Verification items for the finished model (mm, model axes). A direction names the side the tool comes from. Give positions to 0.01 mm unless a question says otherwise; leave off trailing zeros. Write each loop counter-clockwise with the first axis right and the second up, starting at its lowest first coordinate (ties: lowest second). Pieces come first, ordered by that corner, then holes. Notation, with made-up numbers: M 87.25,10.5 L 144.25,10.5 A16 cw 144.25,25.5 Z; hole C -16.5,54 d11. An arc over 180 degrees is marked long. Answer as a JSON object with one key per item and string values.
```python
from build123d import *

# Parameters (mm, degrees)
CROQUIS1_W              = 55.5
CROQUIS1_H              = 20
CROQUIS1_R              = 1.000000224
CROQUIS1_R_2            = 1.000000066
CROQUIS1_R_3            = 1.500000028
CROQUIS1_R_4            = 0.999999891
CROQUIS1_R_5            = 0.999999587
CROQUIS1_W_2            = 15
CROQUIS1_H_2            = 10
SALIENTE_EXTRUIR1_DEPTH = 4.1
CROQUIS2_W              = 42
CROQUIS2_H              = 20
CROQUIS2_R              = 1.500000028
CROQUIS2_W_2            = 15
CROQUIS2_H_2            = 10
SALIENTE_EXTRUIR2_DEPTH = 5.4
CROQUIS3_R              = 10.033223334
CROQUIS3_R_2            = 1.500000028
SALIENTE_EXTRUIR3_DEPTH = 3.5
CROQUIS4_R              = 5
CROQUIS4_R_2            = 1.500000028
SALIENTE_EXTRUIR4_DEPTH = 3.4


with BuildPart() as part:
    # Croquis1 → Saliente-Extruir1 (new body)
    with BuildSketch(Plane(origin=(0, 0, 0), x_dir=(1, 0, 0), z_dir=(0, 1, 0))):
        with Locations((-0.49546198, -0.123865495)):
            Rectangle(CROQUIS1_W, CROQUIS1_H)
        with Locations((-24.995460911, 4.876134086)):
            Circle(CROQUIS1_R, mode=Mode.SUBTRACT)
        with Locations((-24.995461734, -5.123865495)):
            Circle(CROQUIS1_R_2, mode=Mode.SUBTRACT)
        with Locations((9.504538064, -0.123865505)):
            Circle(CROQUIS1_R_3, mode=Mode.SUBTRACT)
        with Locations((24.004538739, 4.876134747)):
            Circle(CROQUIS1_R_4, mode=Mode.SUBTRACT)
        with Locations((24.004537606, -5.123865416)):
            Circle(CROQUIS1_R_5, mode=Mode.SUBTRACT)
        with Locations((-9.99546198, -0.123865495)):
            Rectangle(CROQUIS1_W_2, CROQUIS1_H_2, mode=Mode.SUBTRACT)
    extrude(amount=SALIENTE_EXTRUIR1_DEPTH)

    # Croquis2 → Saliente-Extruir2 (add)
    with BuildSketch(Plane(origin=(0, 4.1, 0), x_dir=(1, 0, 0), z_dir=(0, 1, 0))):
        with Locations((-0.49546198, -0.123865495)):
            Rectangle(CROQUIS2_W, CROQUIS2_H)
        with Locations((9.504538064, -0.123865505)):
            Circle(CROQUIS2_R, mode=Mode.SUBTRACT)
        with Locations((-9.99546198, -0.123865495)):
            Rectangle(CROQUIS2_W_2, CROQUIS2_H_2, mode=Mode.SUBTRACT)
    extrude(amount=SALIENTE_EXTRUIR2_DEPTH)

    # Croquis3 → Saliente-Extruir3 (add)
    with BuildSketch(Plane(origin=(0, 9.5, 0), x_dir=(1, 0, 0), z_dir=(0, 1, 0))):
        with Locations((9.504538064, -0.123865505)):
            Circle(CROQUIS3_R)
        with Locations((9.504538064, -0.123865505)):
            Circle(CROQUIS3_R_2, mode=Mode.SUBTRACT)
    extrude(amount=SALIENTE_EXTRUIR3_DEPTH)

    # Croquis4 → Saliente-Extruir4 (add)
    with BuildSketch(Plane(origin=(0, 13, 0), x_dir=(1, 0, 0), z_dir=(0, 1, 0))):
        with Locations((9.504538064, -0.123865505)):
            Circle(CROQUIS4_R)
        with Locations((9.504538064, -0.123865505)):
            Circle(CROQUIS4_R_2, mode=Mode.SUBTRACT)
    extrude(amount=SALIENTE_EXTRUIR4_DEPTH)


solid = part.part
```
1) Section check C-C on y = 3.5. Record the boundary of the cut face in (x, z), and give its area (3 significant figures).
Completed:
{"outline": "M -28.25,-9.88 L 27.25,-9.88 L 27.25,10.12 L -28.25,10.12 Z; hole C -25,-4.88 d2; hole C -25,5.12 d2; hole M -17.5,-4.88 L -2.5,-4.88 L -2.5,5.12 L -17.5,5.12 Z; hole C 9.5,0.12 d3; hole C 24,-4.88 d2; hole C 24,5.12 d2", "area": "940 mm2"}
2) Access from +Z, -Z, +X, -X, +Y, -Y to the whole of each face (thin tool, end or side, straight path). Record for faces 4 (the face through (-17.495, 5, 0)), 5 (the face through (24, 4.1, 0)), 6 (the face through (7.1, 13, -4.5)).
Completed:
{"face 4": "+Y, -Y", "face 5": "+Z, -Z, +X, +Y", "face 6": "+Y"}
3) Go/stop test with flat-tipped pins: pin 1 (5 mm diameter, centred on x = -20.5, z = 5, fed in from +Y); pin 2 (3 mm diameter, centred on x = -7, z = -7.5, fed in from -Y); pin 3 (5 mm diameter, centred on x = 2.5, y = 3.5, fed in from -Z); pin 4 (10 mm diameter, centred on x = -5, z = -0.5, fed in from +Y). Record where each tip stops, or that it passes through.
Completed:
{"pin 1": "stops at y = 9.5", "pin 2": "stops at y = 0", "pin 3": "stops at z = -9.88", "pin 4": "stops at y = 13"}
4) Thickness scan on L1, parallel to Z at x = 24, y = 3.75; L2, parallel to X at y = 8.5, z = 4.5; L3, parallel to X at y = 2, z = 2. Record the ranges inside material, lowest first.
Completed:
{"L1": "z = -9.88 to -5.88, -3.88 to 4.12, 6.12 to 10.12", "L2": "x = -21.5 to -17.5, -2.5 to 20.5", "L3": "x = -28.25 to -17.5, -2.5 to 27.25"}
5) Release check for a two-part mould opening along X. For faces 1 (the face through (20.505, 7, 0)), 2 (the face through (-1, 5, -9.876)), 3 (the face through (24.958, 2.021, -5.177)) record: pulls with the +X half, pulls with the -X half, needs draft (parallel to the pull), parting line crosses it, or undercut.
Completed:
{"face 1": "pulls with the +X half", "face 2": "needs draft", "face 3": "undercut"}
6) Section check D-D on z = -7.25. Record the boundary of the cut face in (x, y), and give its area (3 significant figures).
Completed:
{"outline": "M -28.25,0 L 27.25,0 L 27.25,4.1 L 20.5,4.1 L 20.5,9.5 L 16.31,9.5 L 16.31,13 L 2.7,13 L 2.7,9.5 L -21.5,9.5 L -21.5,4.1 L -28.25,4.1 Z", "area": "502 mm2"}
7) Section check B-B on z = -2. Record the boundary of the cut face in (x, y), and give its area (3 significant figures).
Completed:
{"outline": "M -28.25,0 L -17.5,0 L -17.5,9.5 L -21.5,9.5 L -21.5,4.1 L -28.25,4.1 Z; M -2.5,0 L 27.25,0 L 27.25,4.1 L 20.5,4.1 L 20.5,9.5 L 19.31,9.5 L 19.31,13 L 14.03,13 L 14.03,16.4 L 4.98,16.4 L 4.98,13 L -0.3,13 L -0.3,9.5 L -2.5,9.5 Z", "area": "411 mm2"}
8) Section check A-A on x = -7. Record the boundary of the cut face in (y, z).
Completed:
{"outline": "M 0,-9.88 L 9.5,-9.88 L 9.5,-4.88 L 0,-4.88 Z; M 0,5.12 L 9.5,5.12 L 9.5,10.12 L 0,10.12 Z"}
